```python
from build123d import *

# Parameters (mm, degrees)
F1_DEPTH = 12.7
F0_R     = 6.573501
F2_DEPTH = 31.496


with BuildPart() as f1:
    # F0 (on Front) → F1 (new body)
    with BuildSketch(Plane.XZ):
        with BuildLine():
            Line((-37.489949, -17.095566), (29.513806, -17.095566))
            ThreePointArc((29.513806, -17.095566), (12.41824, 0), (29.513806, 17.095566))
            Line((29.513806, 17.095566), (-37.489949, 17.095566))
            Line((-37.489949, 17.095566), (-37.489949, 6.573501))
            ThreePointArc((-37.489949, 6.573501), (-32.841781, 4.648167), (-30.916447, 0))
            ThreePointArc((-30.916447, 0), (-32.841781, -4.648167), (-37.489949, -6.573501))
            Line((-37.489949, -6.573501), (-37.489949, -17.095566))
        make_face()
        with BuildLine():
            ThreePointArc((-37.489949, 17.095566), (-54.585515, 0), (-37.489949, -17.095566))
            Line((-37.489949, -17.095566), (-37.489949, -6.573501))
            ThreePointArc((-37.489949, -6.573501), (-44.06345, 0), (-37.489949, 6.573501))
            Line((-37.489949, 6.573501), (-37.489949, 17.095566))
        make_face()
    extrude(amount=-F1_DEPTH)

    # F0 (on Front) → F2 (join)
    with BuildSketch(Plane.XZ):
        with BuildLine():
            ThreePointArc((29.513806, 17.095566), (12.41824, 0), (29.513806, -17.095566))
            ThreePointArc((29.513806, -17.095566), (46.609372, 0), (29.513806, 17.095566))
        make_face()
        with Locations((29.513806, 0)):
            Circle(F0_R, mode=Mode.SUBTRACT)
    extrude(amount=-F2_DEPTH)

    # F3: F1 across face


with BuildPart() as f1_1:
    add(f1.part)
    add(f1.part.mirror(Plane(origin=(29.513806, 31.496, 0), x_dir=(1, 0, 0), z_dir=(0, 1, 0))))


solid = f1_1.part
```
Read the model definition and answer for the solid it produces. Units are mm, in the model's axes. Give positions to 0.01 mm unless a question says otherwise; leave off trailing zeros. Loops run counter-clockwise (first coordinate to the right, second up) from the corner with the lowest first, then second, coordinate; pieces in that order, holes last.
Item 1: The part is cut by section B-B (z = -2). Write down the section's boundary in (x, y).
Item 2: Each of these flat-tipped pins is pushed along its axis until it touches: pin 1 Ø4 at (y, z) = (8, 4) entering from +X; pin 2 Ø1 at (y, z) = (18, 0.5) entering from -X; pin 3 Ø1 at (y, z) = (43.5, -2) entering from -X. Where does it stop, or does it pass through?
Item 3: The part is cut by section D-D (y = 41.5). Write down the section's boundary in (x, z).
Item 4: The part is cut by section C-C (y = 7). Write down the section's boundary in (x, z), and give its area (3 significant figures).
Item 5: The part is cut by section A-A (x = -26.5). Write down the section's boundary in (y, z), and give its area (3 significant figures).
Item 6: Find the intervals of material crossed by line 1 along Y through (x, z) = (-4.5, 2); line 2 along X through (y, z) = (57, 2); line 3 along X through (y, z) = (3, -6), in increasing order.
Item 7: The mould has two halves that part along Y. Classify faces 1 (the flat face through (-13, 12.7, 0)), 2 (the flat face through (-5, 0, 0)), 3 (the flat face through (-4, 6, 17.096)): released by +Y, released by -Y, zero draft, split by the parting line, or undercut.
Taken from the geometry:
1. outline: (-54.47, 0) - (-43.75, 0) - (-43.75, 12.7) - (-54.47, 12.7) - close; (-54.47, 50.29) - (-43.75, 50.29) - (-43.75, 62.99) - (-54.47, 62.99) - close; (-31.23, 0) - (23.25, 0) - (23.25, 62.99) - (-31.23, 62.99) - (-31.23, 50.29) - (12.54, 50.29) - (12.54, 12.7) - (-31.23, 12.7) - close; (35.78, 0) - (46.49, 0) - (46.49, 62.99) - (35.78, 62.99) - close
2. pin 1: stops at x = 46.49
2. pin 2: stops at x = 12.42
2. pin 3: stops at x = 12.48
3. outline: circle Ø34.19 at (29.51, 0); hole circle Ø13.15 at (29.51, 0)
4. outline: (-37.49, -17.1) - (29.51, -17.1) arc R17.1 ccw to (29.51, 17.1) - (-37.49, 17.1) arc R17.1 ccw to start; hole circle Ø13.15 at (-37.49, 0); hole circle Ø13.15 at (29.51, 0)
4. area: 2,940 mm2
5. outline: (0, -17.1) - (12.7, -17.1) - (12.7, 17.1) - (0, 17.1) - close; (50.29, -17.1) - (62.99, -17.1) - (62.99, 17.1) - (50.29, 17.1) - close
5. area: 868 mm2
6. line 1: y = 0 to 12.7, 50.29 to 62.99
6. line 2: x = -54.47 to -43.75, -31.23 to 23.25, 35.78 to 46.49
6. line 3: x = -53.5 to -40.18, -34.8 to 26.83, 32.2 to 45.52
7. face 1: undercut
7. face 2: released by -Y
7. face 3: zero draft
